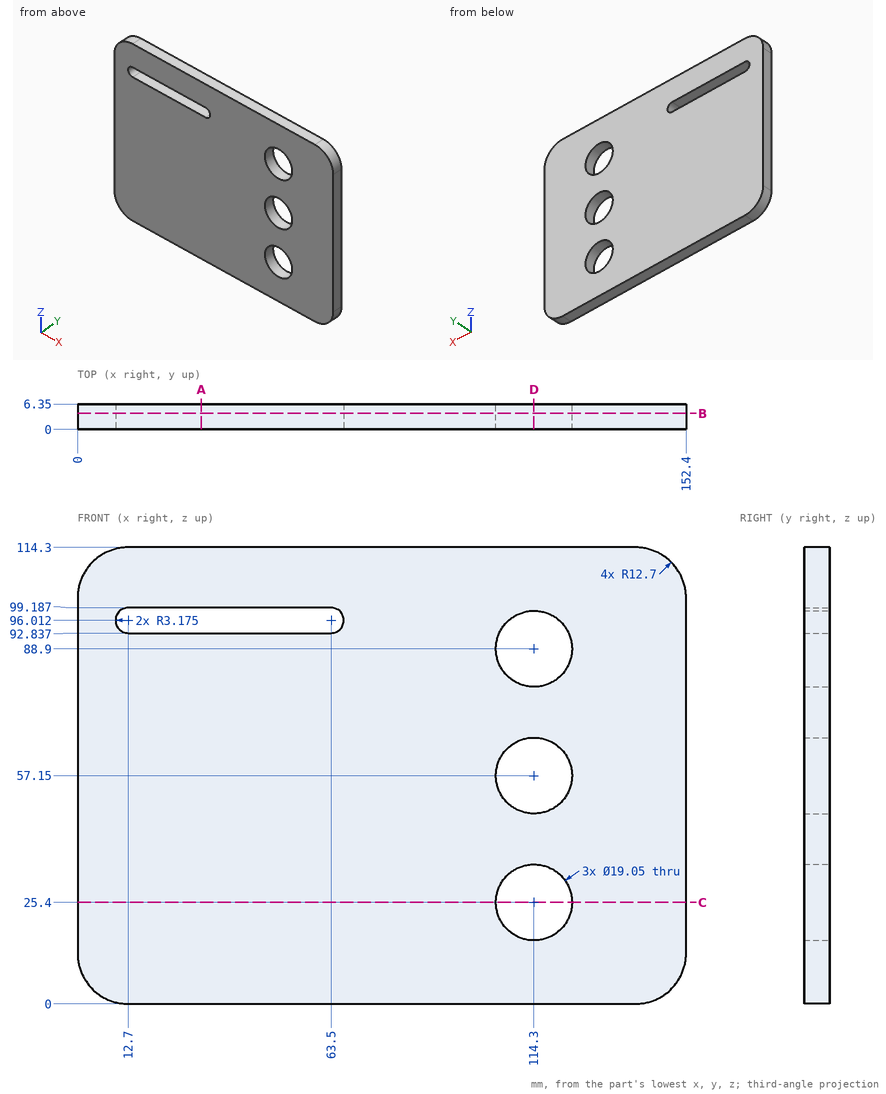
Input: dimensioned drawing with shaded views. Units: mm. Origin: part minimum x, y, z. Give positions to 0.01 mm unless a question says otherwise; leave off trailing zeros. Loops run counter-clockwise (first coordinate to the right, second up) from the corner with the lowest first, then second, coordinate; pieces in that order, holes last. Notation, with made-up numbers: (46.5, 13) -> (70.5, 13) arc R21 cw to (70.5, 28) -> close; hole circle Ø1 at (71, 85). An arc over 180 degrees is marked (long way). Use a Markdown table: item, result. Add a question column.
1) First-contact query: pin 1 (2 mm diameter, centred on y = 5.5, z = 12, fed in from +X). Flat tip, straight axial feed; report the tip coordinate or a pass-through.
2) Section query A-A, the plane x = 31. Return the cut outline in (y, z), then the cut area to 3 significant figures.
3) Section query C-C, the plane z = 25.4. Return the cut outline in (x, y) (3 decimals).
4) Line query: line 1 along Z through (x, y) = (114.3, 5) (3 decimals); line 2 along Z through (x, y) = (59, 4); line 3 along X through (y, z) = (0.5, 25). Output: solid intervals per line, ascending. Write a range as [from, to].
5) Section query D-D, the plane x = 114.3. Return the cut outline in (y, z) (3 decimals).
6) Section query B-B, the plane y = 4. Return the cut outline in (x, z) (3 decimals), then the cut area to 3 significant figures.
Numbers:
| question | item | result |
|---|---|---|
| 1 | pin 1 | stops at x = 152.4 |
| 2 | outline | (0, 0) -> (6.35, 0) -> (6.35, 92.84) -> (0, 92.84) -> close; (0, 99.19) -> (6.35, 99.19) -> (6.35, 114.3) -> (0, 114.3) -> close |
| 2 | area | 685 mm2 |
| 3 | outline | (0, 0) -> (104.775, 0) -> (104.775, 6.35) -> (0, 6.35) -> close; (123.825, 0) -> (152.4, 0) -> (152.4, 6.35) -> (123.825, 6.35) -> close |
| 4 | line 1 | z = [0, 15.875], [34.925, 47.625], [66.675, 79.375], [98.425, 114.3] |
| 4 | line 2 | z = [0, 92.84], [99.19, 114.3] |
| 4 | line 3 | x = [0, 104.78], [123.82, 152.4] |
| 5 | outline | (0, 0) -> (6.35, 0) -> (6.35, 15.875) -> (0, 15.875) -> close; (0, 34.925) -> (6.35, 34.925) -> (6.35, 47.625) -> (0, 47.625) -> close; (0, 66.675) -> (6.35, 66.675) -> (6.35, 79.375) -> (0, 79.375) -> close; (0, 98.425) -> (6.35, 98.425) -> (6.35, 114.3) -> (0, 114.3) -> close |
| 6 | outline | (0, 12.7) arc R12.7 ccw to (12.7, 0) -> (139.7, 0) arc R12.7 ccw to (152.4, 12.7) -> (152.4, 101.6) arc R12.7 ccw to (139.7, 114.3) -> (12.7, 114.3) arc R12.7 ccw to (0, 101.6) -> close; hole (12.7, 92.837) -> (63.5, 92.837) arc R3.175 ccw to (63.5, 99.187) -> (12.7, 99.187) arc R3.175 ccw to start; hole circle Ø19.05 at (114.3, 25.4); hole circle Ø19.05 at (114.3, 57.15); hole circle Ø19.05 at (114.3, 88.9) |
| 6 | area | 16,100 mm2 |
